Design review of the part built by this model. Coordinates are the model's own, in mm. Give positions to 0.01 mm unless a question says otherwise; leave off trailing zeros. Loops run counter-clockwise (first coordinate to the right, second up) from the corner with the lowest first, then second, coordinate; pieces in that order, holes last. Notation, with made-up numbers: (-32.75, 31.25) -> (-16.75, 31.25) arc R12 cw to (-16.75, 40.25) -> close; hole circle Ø10 at (-7, 64). An arc over 180 degrees is marked (long way). Use CSV: the item, a comma, the result in double quotes. Start each with the question number.
Item 1: We need section A-A (y = 0.8). State the section outline as (x, z) points, plus the area to 3 significant figures.
Item 2: Clearance check with a flat-ended pin moving along its axis: pin 1 (2.5 mm diameter, centred on x = -15, z = 0, fed in from +Y). State where the tip first meets the part, or that it passes through.
Item 3: We need section C-C (z = -2.4). State the section outline as (x, y) points, plus the area to 3 significant figures.
Item 4: The part is to be moulded in two halves that separate along Z. For faces 1 (the face through (0, 1, -2)), 2 (the face through (0, 1, 2)), 3 (the face through (-13.562, 1.014, -0.189)), say which applies: +Z half, -Z half, draft (parallel to the pull), parting line (faces both ways), or undercut.
Item 5: We need section D-D (x = -6). State the section outline as (y, z) points, plus the area to 3 significant figures.
Item 6: We need section B-B (z = 0). State the section outline as (x, y) points.
Item 7: Wall thickness on line 1 along X through (y, z) = (0.7, 0); line 2 along X through (y, z) = (1.15, -0.85); line 3 along Z through (x, y) = (-2.5, 0.3): over which ranges is each line inside the solid? List them lowest first. Write a range as from..to.
from build123d import *

# Parameters (mm, degrees)
SALIENTE_EXTRUIR1_DEPTH = 2
CROQUIS_BARRENOS_R      = 1.45
CORTAR_EXTRUIR1_DEPTH   = 2


with BuildPart() as part:
    # Croquis base → Saliente-Extruir1 (new body)
    with BuildSketch(Plane(origin=(0, 0, 0), x_dir=(1, 0, 0), z_dir=(0, 1, 0))):
        with BuildLine():
            Line((12.763932023, 2), (-12.763932023, 2))
            ThreePointArc((-12.763932023, 2), (-13.775255129, 2.738612788), (-15, 3))
            ThreePointArc((-15, 3), (-18, 0), (-15, -3))
            ThreePointArc((-15, -3), (-13.775255129, -2.738612788), (-12.763932023, -2))
            Line((-12.763932023, -2), (12.763932023, -2))
            ThreePointArc((12.763932023, -2), (13.775255129, -2.738612788), (15, -3))
            ThreePointArc((15, -3), (18, 0), (15, 3))
            ThreePointArc((15, 3), (13.775255129, 2.738612788), (12.763932023, 2))
        make_face()
    extrude(amount=SALIENTE_EXTRUIR1_DEPTH)

    # Croquis barrenos → Cortar-Extruir1 (cut)
    with BuildSketch(Plane(origin=(0, 2, 0), x_dir=(1, 0, 0), z_dir=(0, 1, 0))):
        with Locations(Location((-15, 0, 0), (0, 0, 270))):
            Circle(CROQUIS_BARRENOS_R)
        with Locations(Location((15, 0, 0), (0, 0, 270))):
            Circle(CROQUIS_BARRENOS_R)
    extrude(amount=-CORTAR_EXTRUIR1_DEPTH, mode=Mode.SUBTRACT)


solid = part.part
Results found:
1,outline,"(-12.76, -2) -> (12.76, -2) arc R3 ccw (long way) to (12.76, 2) -> (-12.76, 2) arc R3 ccw (long way) to start; hole circle Ø2.9 at (-15, 0); hole circle Ø2.9 at (15, 0)"
1,area,"141 mm²"
2,pin 1,"through"
3,outline,"(-16.8, 0) -> (-13.2, 0) -> (-13.2, 2) -> (-16.8, 2) -> close; (13.2, 0) -> (16.8, 0) -> (16.8, 2) -> (13.2, 2) -> close"
3,area,"14.4 mm²"
4,face 1,"-Z half"
4,face 2,"+Z half"
4,face 3,"undercut"
5,outline,"(0, -2) -> (2, -2) -> (2, 2) -> (0, 2) -> close"
5,area,"8.00 mm²"
6,outline,"(-18, 0) -> (-16.45, 0) -> (-16.45, 2) -> (-18, 2) -> close; (-13.55, 0) -> (13.55, 0) -> (13.55, 2) -> (-13.55, 2) -> close; (16.45, 0) -> (18, 0) -> (18, 2) -> (16.45, 2) -> close"
7,line 1,"-18..-16.45, -13.55..13.55, 16.45..18"
7,line 2,"-17.88..-16.17, -13.83..13.83, 16.17..17.88"
7,line 3,"-2..2"
